```python
from build123d import *

# Parameters (mm, degrees)
SKETCH1_R                              = 87.5
BOSS_EXTRUDE1_DEPTH                    = 10
SKETCH2_R                              = 7.5
BOSS_EXTRUDE2_DEPTH                    = 80
CBORE_FOR_M5_HEX_HEAD_BOLT1_AT_2_COUNT = 2
CBORE_FOR_M5_HEX_HEAD_BOLT1_AT_2_PITCH = 113.13708499
CBORE_FOR_M5_HEX_HEAD_BOLT1_AT_3_COUNT = 2
CBORE_FOR_M5_HEX_HEAD_BOLT1_AT_3_PITCH = 160
CBORE_FOR_M5_HEX_HEAD_BOLT1_AT_4_COUNT = 2
CBORE_FOR_M5_HEX_HEAD_BOLT1_AT_4_PITCH = 113.13708499
SKETCH5_R                              = 87.5
CUT_EXTRUDE1_DEPTH                     = 80
FILLET1_R                              = 0.1
SKETCH6_R                              = 5
BOSS_EXTRUDE3_DEPTH                    = 5
BOSS_EXTRUDE3_TAPER                    = 30
SKETCH7_R                              = 1.45
CUT_EXTRUDE2_DEPTH                     = 8
SKETCH9_R                              = 5
CUT_EXTRUDE3_DEPTH                     = 10
CUT_EXTRUDE5_DEPTH                     = 10
CBORE_FOR_M5_HEX_HEAD_BOLT2_AT_2_COUNT = 2
CBORE_FOR_M5_HEX_HEAD_BOLT2_AT_2_PITCH = 120


with BuildPart() as part:
    # Sketch1 → Boss-Extrude1 (new body)
    with BuildSketch(Plane(origin=(0, 0, 0), x_dir=(1, 0, 0), z_dir=(0, 1, 0))):
        Circle(SKETCH1_R)
    extrude(amount=BOSS_EXTRUDE1_DEPTH)

    # Sketch2 → Boss-Extrude2 (add)
    with BuildSketch(Plane(origin=(0, 10, 0), x_dir=(1, 0, 0), z_dir=(0, 1, 0))):
        with Locations((0, -80)):
            Circle(SKETCH2_R)
        with Locations((-80, 0)):
            Circle(SKETCH2_R)
        with Locations((0, 80)):
            Circle(SKETCH2_R)
        with Locations((80, 0)):
            Circle(SKETCH2_R)
    extrude(amount=BOSS_EXTRUDE2_DEPTH)

    # Sketch4 → CBORE for M5 Hex Head Bolt1 (revolve, cut)
    with BuildSketch(Plane(origin=(80, 0, 0), x_dir=(0, 0, -1), z_dir=(1, 0, 0))):
        Polygon((0, 0), (0, 21.652366702), (2.75, 20), (2.75, 3.58), (6.12, 3.58), (6.12, 0.025), (6.145, 0), align=None)
    cbore_for_m5_hex_head_bolt1 = revolve(axis=Axis((80, -6.35, 0), (0, 1, 0)), mode=Mode.SUBTRACT)

    # CBORE for M5 Hex Head Bolt1 at 2: CBORE for M5 Hex Head Bolt1 ×2
    with Locations(*[Vector(-0.707106781, 0, -0.707106781) * (i * CBORE_FOR_M5_HEX_HEAD_BOLT1_AT_2_PITCH) for i in range(1, CBORE_FOR_M5_HEX_HEAD_BOLT1_AT_2_COUNT)]):
        add(cbore_for_m5_hex_head_bolt1, mode=Mode.SUBTRACT)

    # CBORE for M5 Hex Head Bolt1 at 3: CBORE for M5 Hex Head Bolt1 ×2
    with Locations(*[(-i * CBORE_FOR_M5_HEX_HEAD_BOLT1_AT_3_PITCH, 0, 0) for i in range(1, CBORE_FOR_M5_HEX_HEAD_BOLT1_AT_3_COUNT)]):
        add(cbore_for_m5_hex_head_bolt1, mode=Mode.SUBTRACT)

    # CBORE for M5 Hex Head Bolt1 at 4: CBORE for M5 Hex Head Bolt1 ×2
    with Locations(*[Vector(-0.707106781, 0, 0.707106781) * (i * CBORE_FOR_M5_HEX_HEAD_BOLT1_AT_4_PITCH) for i in range(1, CBORE_FOR_M5_HEX_HEAD_BOLT1_AT_4_COUNT)]):
        add(cbore_for_m5_hex_head_bolt1, mode=Mode.SUBTRACT)

    # Sketch5 → Cut-Extrude1 (cut)
    with BuildSketch(Plane(origin=(0, 10, 0), x_dir=(1, 0, 0), z_dir=(0, 1, 0))):
        Circle(SKETCH5_R)
    extrude(amount=CUT_EXTRUDE1_DEPTH, mode=Mode.SUBTRACT)

    # Fillet1
    fillet1_edges = [part.edges().sort_by_distance(p)[0] for p in [
        (-87.5, 0, 0),
    ]]
    fillet(fillet1_edges, radius=FILLET1_R)

    # Sketch6 → Boss-Extrude3 (add)
    with BuildSketch(Plane(origin=(0, 10, 0), x_dir=(1, 0, 0), z_dir=(0, 1, 0))):
        with Locations((-15.25, 15.25)):
            Circle(SKETCH6_R)
        with Locations((15.25, 15.25)):
            Circle(SKETCH6_R)
        with Locations((15.25, -15.25)):
            Circle(SKETCH6_R)
        with Locations((-15.25, -15.25)):
            Circle(SKETCH6_R)
    extrude(amount=BOSS_EXTRUDE3_DEPTH, taper=BOSS_EXTRUDE3_TAPER)

    # Sketch7 → Cut-Extrude2 (cut)
    with BuildSketch(Plane(origin=(0, 15, 0), x_dir=(1, 0, 0), z_dir=(0, 1, 0))):
        with Locations((-15.25, 15.25)):
            Circle(SKETCH7_R)
        with Locations((15.25, 15.25)):
            Circle(SKETCH7_R)
        with Locations((15.25, -15.25)):
            Circle(SKETCH7_R)
        with Locations((-15.25, -15.25)):
            Circle(SKETCH7_R)
    extrude(amount=-CUT_EXTRUDE2_DEPTH, mode=Mode.SUBTRACT)

    # Sketch9 → Cut-Extrude3 (cut)
    with BuildSketch(Plane.XZ):
        with Locations((38.003300859, 60.053300859)):
            Circle(SKETCH9_R)
        with Locations((-35.303300859, 60.053300859)):
            Circle(SKETCH9_R)
        with Locations((-35.303300859, -64.053300859)):
            Circle(SKETCH9_R)
        with Locations((38.003300859, -64.053300859)):
            Circle(SKETCH9_R)
    extrude(amount=-CUT_EXTRUDE3_DEPTH, mode=Mode.SUBTRACT)

    # Sketch10 → Cut-Extrude5 (cut)
    with BuildSketch(Plane.XZ):
        with BuildLine():
            Line((-86.336119643, -14.224079762), (-46.336119643, -14.224079762))
            Line((-46.336119643, -14.224079762), (-46.336119643, -74.224079762))
            ThreePointArc((-46.336119643, -74.224079762), (-72.804400755, -48.53626717), (-86.336119643, -14.224079762))
        make_face()
        with BuildLine():
            Line((-46.336119643, 14.224079762), (-46.336119643, 74.224079762))
            ThreePointArc((-46.336119643, 74.224079762), (-72.804400755, 48.53626717), (-86.336119643, 14.224079762))
            Line((-86.336119643, 14.224079762), (-46.336119643, 14.224079762))
        make_face()
        with BuildLine():
            Line((46.336119643, 14.224079762), (86.336119643, 14.224079762))
            ThreePointArc((86.336119643, 14.224079762), (72.804400755, 48.53626717), (46.336119643, 74.224079762))
            Line((46.336119643, 74.224079762), (46.336119643, 14.224079762))
        make_face()
        with BuildLine():
            Line((46.336119643, -14.224079762), (46.336119643, -74.224079762))
            ThreePointArc((46.336119643, -74.224079762), (72.804400755, -48.53626717), (86.336119643, -14.224079762))
            Line((86.336119643, -14.224079762), (46.336119643, -14.224079762))
        make_face()
    extrude(amount=-CUT_EXTRUDE5_DEPTH, mode=Mode.SUBTRACT)

    # Sketch13 → CBORE for M5 Hex Head Bolt2 (revolve, cut)
    with BuildSketch(Plane(origin=(-60, 10, 0), x_dir=(0, 0, 1), z_dir=(1, 0, 0))):
        Polygon((0, 0), (0, 10), (2.75, 10), (2.75, 3.58), (6.12, 3.58), (6.12, 0.025), (6.145, 0), align=None)
    cbore_for_m5_hex_head_bolt2 = revolve(axis=Axis((-60, 16.35, 0), (0, -1, 0)), mode=Mode.SUBTRACT)

    # CBORE for M5 Hex Head Bolt2 at 2: CBORE for M5 Hex Head Bolt2 ×2
    with Locations(*[(i * CBORE_FOR_M5_HEX_HEAD_BOLT2_AT_2_PITCH, 0, 0) for i in range(1, CBORE_FOR_M5_HEX_HEAD_BOLT2_AT_2_COUNT)]):
        add(cbore_for_m5_hex_head_bolt2, mode=Mode.SUBTRACT)


solid = part.part
```
Verification items for the finished model (mm, model axes). A direction names the side the tool comes from. Coordinates: 2 decimals unless noted, no trailing zeros. Loops run counter-clockwise (first coordinate to the right, second up) from the corner with the lowest first, then second, coordinate; pieces in that order, holes last. Notation, with made-up numbers: (72.5, 82) -> (84.5, 82) arc R6 cw to (84.5, 93) -> close; hole circle Ø9 at (32.5, 0). An arc over 180 degrees is marked (long way). Answer in a Markdown table with one row per item.
1) Section check C-C (y = 12). Record the cut outline in (x, z).
The answers:
| item | result |
|---|---|
| outline | circle Ø7.69 at (-15.25, -15.25); circle Ø7.69 at (-15.25, 15.25); circle Ø7.69 at (15.25, -15.25); circle Ø7.69 at (15.25, 15.25); hole circle Ø2.9 at (-15.25, -15.25); hole circle Ø2.9 at (-15.25, 15.25); hole circle Ø2.9 at (15.25, -15.25); hole circle Ø2.9 at (15.25, 15.25) |
2) Draft check along X on faces 1 (the face through (57.273, 3.255, -0.358)), 2 (the face through (66, 5, 14.224)), 3 (the face through (-46.336, 5, -44)), 4 (the face through (-79, 3.58, 3)). Enter one of: released by +X, released by -X, zero draft, split by the parting line, or undercut.
The answers:
| item | result |
|---|---|
| face 1 | undercut |
| face 2 | zero draft |
| face 3 | released by -X |
| face 4 | undercut |
3) Section check D-D (z = 0). Give the number of separate pieces and of enclosed holes in the cut face, and give its area (3 significant figures).
The answers:
| item | result |
|---|---|
| separate pieces | 5 |
| enclosed holes | 0 |
| area | 1,430 mm2 |
4) Scan lines: line 1 along Z through (x, y) = (-15.25, 9.75); line 2 along X through (y, z) = (4.5, 0); line 3 along Z through (x, y) = (-3.5, 1.5). Record each from-to range of solid material in increasing order. Write a range as from..to.
The answers:
| item | result |
|---|---|
| line 1 | z = -86.16..-16.7, -13.8..13.8, 16.7..86.16 |
| line 2 | x = -87.5..-82.75, -77.25..-62.75, -57.25..57.25, 62.75..77.25, 82.75..87.5 |
| line 3 | z = -87.43..-85.02, -74.98..74.98, 85.02..87.43 |
5) Depth check by flat-ended pin: P1, Ø1.5, axis at x = -18, y = 9.5, coming from the +Z side; P2, Ø6.5, axis at x = 60, z = 0, coming from the +Y side; P3, Ø10, axis at x = 57.5, z = 0, coming from the +Y side. Enter the tip coordinate at first touch or a pass-through.
The answers:
| item | result |
|---|---|
| P1 | stops at z = 85.78 |
| P2 | stops at y = 6.42 |
| P3 | stops at y = 10 |
6) Access from +Z, -Z, +X, -X, +Y, -Y to the whole of each face (thin tool, end or side, straight path). Record for faces 5 (the face through (34.035, 4.93, 57.011)), 6 (the face through (81, 3.58, 3)).
The answers:
| item | result |
|---|---|
| face 5 | +Y, -Y |
| face 6 | -Y |
7) Section check B-B (x = 80). Record the cut outline in (y, z) (3 decimals), and give its area (3 significant figures).
The answers:
| item | result |
|---|---|
| outline | (0, -14.224) -> (10, -14.224) -> (10, -2.75) -> (3.58, -2.75) -> (3.58, -6.12) -> (0.025, -6.12) -> (0, -6.145) -> close; (0, 6.145) -> (0.025, 6.12) -> (3.58, 6.12) -> (3.58, 2.75) -> (10, 2.75) -> (10, 14.224) -> (0, 14.224) -> close |
| area | 205 mm2 |
8) Section check A-A (x = 0). Record the cut outline in (y, z) (3 decimals).
The answers:
| item | result |
|---|---|
| outline | (0, -87.4) arc R0.1 ccw to (0.1, -87.5) -> (10, -87.5) -> (10, -82.75) -> (3.58, -82.75) -> (3.58, -86.12) -> (0.025, -86.12) -> (0, -86.145) -> close; (0, -73.855) -> (0.025, -73.88) -> (3.58, -73.88) -> (3.58, -77.25) -> (10, -77.25) -> (10, 77.25) -> (3.58, 77.25) -> (3.58, 73.88) -> (0.025, 73.88) -> (0, 73.855) -> close; (0, 86.145) -> (0.025, 86.12) -> (3.58, 86.12) -> (3.58, 82.75) -> (10, 82.75) -> (10, 87.5) -> (0.1, 87.5) arc R0.1 ccw to (0, 87.4) -> close |
